from build123d import *

# Parameters (mm, degrees)
F0_W     = 10
F0_H     = 3
F0_W_2   = 32.3
F0_R     = 11.2
F1_DEPTH = 3
F2_DEPTH = 40
F4_DEPTH = 15
F5_DEPTH = 10
F6_SIZE  = 9.99999
F7_R     = 1.6
F8_R     = 1.6
F9_DEPTH = 25


# Not quite as in the source:
# - a fillet or chamfer is up to 0.001 mm smaller than in the source, because OpenCascade refuses the exact size


with BuildPart() as f1:
    # F0 (on Top) → F1 (new body)
    with BuildSketch(Plane.XY):
        Polygon((21.15, -21.15), (21.15, 21.15), (11.15, 21.15), (-21.15, 21.15), (-21.15, -21.15), (11.15, -21.15), align=None)
        with BuildLine():
            ThreePointArc((-16, 14.4), (-17.1313708499, 17.1313708499), (-14.4, 16))
            Line((-14.4, 16), (14.4, 16))
            ThreePointArc((14.4, 16), (16, 17.6), (17.6, 16))
            ThreePointArc((17.6, 16), (17.1313708499, 14.8686291501), (16, 14.4))
            Line((16, 14.4), (16, -14.4))
            ThreePointArc((16, -14.4), (17.1313708499, -14.8686291501), (17.6, -16))
            ThreePointArc((17.6, -16), (16, -17.6), (14.4, -16))
            Line((14.4, -16), (-14.4, -16))
            ThreePointArc((-14.4, -16), (-17.1313708499, -17.1313708499), (-16, -14.4))
            Line((-16, -14.4), (-16, 14.4))
        make_face(mode=Mode.SUBTRACT)
        Polygon((21.15, 24.15), (21.15, 21.15), (21.15, -21.15), (21.15, -24.15), (24.15, -24.15), (24.15, 24.15), align=None)
        with Locations((16.15, 22.65)):
            Rectangle(F0_W, F0_H)
        with Locations((-5, 22.65)):
            Rectangle(F0_W_2, F0_H)
        with Locations((16.15, -22.65)):
            Rectangle(F0_W, F0_H)
        Polygon((11.15, -24.15), (11.15, -21.15), (-21.15, -21.15), (-21.15, -24.15), (9.2402426526, -24.15), align=None)
        with BuildLine():
            Line((14.4, 16), (-14.4, 16))
            ThreePointArc((-14.4, 16), (-14.8686291501, 14.8686291501), (-16, 14.4))
            Line((-16, 14.4), (-16, -14.4))
            ThreePointArc((-16, -14.4), (-14.8686291501, -14.8686291501), (-14.4, -16))
            Line((-14.4, -16), (14.4, -16))
            ThreePointArc((14.4, -16), (14.8686291501, -14.8686291501), (16, -14.4))
            Line((16, -14.4), (16, 14.4))
            ThreePointArc((16, 14.4), (14.8686291501, 14.8686291501), (14.4, 16))
        make_face()
        Circle(F0_R, mode=Mode.SUBTRACT)
    extrude(amount=F1_DEPTH)

    # F0 (on Top) → F2 (join)
    with BuildSketch(Plane.XY):
        Polygon((21.15, 24.15), (21.15, 21.15), (21.15, -21.15), (21.15, -24.15), (24.15, -24.15), (24.15, 24.15), align=None)
    extrude(amount=-F2_DEPTH)

    # F3 (on face) → F4 (join)
    with BuildSketch(Plane.YZ.offset(24.15)):
        Polygon((-0.1639153264, -15.6763265476), (1.329879063, -17.0062056106), (19.1407867495, 3), (16.4630420556, 3), align=None)
        Polygon((19.1407867495, 3), (1.329879063, -17.0062056106), (2.8236734524, -18.3360846736), (21.8185314434, 3), align=None)
        Polygon((1.329879063, -17.0062056106), (0, -18.5), (24.15, -40), (24.15, -37.3222553061), (2.8236734524, -18.3360846736), align=None)
        Polygon((24.15, -40), (0, -18.5), (-1.329879063, -19.9937943894), (21.1422077043, -40), align=None)
        Polygon((0, -18.5), (-24.15, 3), (-24.15, 0.3222553061), (-1.329879063, -19.9937943894), align=None)
        Polygon((-21.1422077043, 3), (-24.15, 3), (0, -18.5), (1.329879063, -17.0062056106), (-0.1639153264, -15.6763265476), align=None)
    extrude(amount=F4_DEPTH)

    # F0 (on Top) → F5 (join)
    with BuildSketch(Plane.XY):
        with Locations((16.15, 22.65)):
            Rectangle(F0_W, F0_H)
        with Locations((16.15, -22.65)):
            Rectangle(F0_W, F0_H)
    extrude(amount=-F5_DEPTH)

    # F6 (size 10 in the source; OpenCascade refuses exactly that, so slightly less here)
    f6_edges = [f1.edges().sort_by_distance(p)[0] for p in [
        (11.15, 22.65, -10),
        (11.15, -22.65, -10),
    ]]
    chamfer(f6_edges, length=F6_SIZE)

    # F7 (on face) + F8 (on face) → F9 (cut)
    with BuildSketch(Plane(origin=(0, -7.8579881454, -8.8265308702), x_dir=(1, 0, 0), z_dir=(0, 0.6649395315, 0.7468971947))):
        with Locations((31.65, 28.5779957713)):
            Circle(F7_R)
    with BuildSketch(Plane(origin=(0, -7.8579881454, -8.8265308702), x_dir=(1, 0, 0), z_dir=(0, 0.6649395315, 0.7468971947))):
        with Locations((31.65, -3.7422464428)):
            Circle(F8_R)
    extrude(amount=-F9_DEPTH, mode=Mode.SUBTRACT)


solid = f1.part
Work out the finished part from the listing and answer in its coordinate system (mm). A direction names the side the tool comes from. Give positions to 0.01 mm unless a question says otherwise; leave off trailing zeros. Write each loop counter-clockwise with the first axis right and the second up, starting at its lowest first coordinate (ties: lowest second). Pieces come first, ordered by that corner, then holes. Notation, with made-up numbers: M -27,31.25 L 5,31.25 A16 cw 5,47.25 Z; hole C 73,-37 d4. An arc over 180 degrees is marked long. Answer as CSV lines item,"result".
Q1. A cutting plane is placed at B-B on y = -4. Write down the section's boundary in (x, z).
A:
outline,"M -21.15,0 L -10.46,0 L -10.46,3 L -21.15,3 Z; M 10.46,0 L 21.15,0 L 21.15,-40 L 24.15,-40 L 24.15,-17.62 L 39.15,-17.62 L 39.15,-12.26 L 24.15,-12.26 L 24.15,3 L 10.46,3 Z"
Q2. The mould has two halves that part along Y. Classify faces 6 (the flat face through (16, -24.15, -4)), 7 (the cylindrical face through (-11.19, 0.49, 1.48)), 8 (the flat face through (-21.15, 0, 1)), 9 (the flat face through (31.545, 12.188, -7.817)): +Y half, -Y half, draft (parallel to the pull), parting line (faces both ways), or undercut.
A:
face 6,"-Y half"
face 7,"undercut"
face 8,"draft"
face 9,"+Y half"
Q3. A cutting plane is placed at D-D on y = 19. Write down the section's boundary in (x, z).
A:
outline,"M -21.15,0 L 21.15,0 L 21.15,-40 L 24.15,-40 L 24.15,-38.09 L 39.15,-38.09 L 39.15,-32.74 L 24.15,-32.74 L 24.15,-0.17 L 39.15,-0.17 L 39.15,3 L -21.15,3 Z"
Q4. A cutting plane is placed at A-A on x = 0. Write down the section's boundary in (y, z), plus the area to 3 significant figures.
A:
outline,"M -24.15,0 L -11.2,0 L -11.2,3 L -24.15,3 Z; M 11.2,0 L 24.15,0 L 24.15,3 L 11.2,3 Z"
area,"77.7 mm²"
Q5. Find the intervals of material crossed by probe 1 along X at (y, z) = (16, 2.35); probe 2 along X at (y, z) = (-16, 0.85); probe 3 along Y at (x, z) = (-16, 1.85), in increasing order. Write a range as [from, to].
A:
probe 1,"x = [-21.15, -17.6], [-14.4, 14.4], [17.6, 39.15]"
probe 2,"x = [-21.15, -17.6], [-14.4, 14.4], [17.6, 24.15]"
probe 3,"y = [-24.15, -17.6], [-14.4, 14.4], [17.6, 24.15]"
Q6. Given P1, Ø12.5, axis at x = 4.5, y = 8.5, coming from the -Z side; P2, Ø10, axis at x = 10.5, z = -10.5, coming from the +Y side; P3, Ø6.5, axis at y = 18, z = -16, coming from the +X side; P4, Ø1, axis at x = 25, z = -4, coming from the +Y side, each flat-ended and moving along its own axis, determine where each tip first touches the part or whether it passes through.
A:
P1,"stops at z = 0"
P2,"passes through"
P3,"stops at x = 24.15"
P4,"stops at y = 16.03"
Q7. A cutting plane is placed at C-C on x = 35. Write down the section's boundary in (y, z), plus the area to 3 significant figures.
A:
outline,"M -24.15,0.32 L 21.14,-40 L 24.15,-40 L 24.15,-37.32 L 2.82,-18.34 L 21.82,3 L 16.46,3 L -0.16,-15.68 L -21.14,3 L -24.15,3 Z"
area,"358 mm²"
Q8. A tool of negligible diameter and unlimited length cuts with its end or side. For faces 1 (the flat face through (24.15, -3, -2)), 2 (the flat face through (29.878, 13.636, -27.962)), 3 (the cylindrical face through (33.176, 12.535, -29.622)), 4 (the flat face through (17, 21.15, -4)), 5 (the flat face through (24.15, -12, -29)), from which of +Z, -Z, +X, -X, +Y, -Y can it reach the whole face along a straight path? Write none if from no direction.
A:
face 1,"+Z, +X"
face 2,"+X, +Y"
face 3,"none"
face 4,"-Z, -X"
face 5,"-Z, +X, -Y"
